Geometry check sheet. Reference: the model listing, model coordinates, mm. A direction names the side the tool comes from. Round coordinates to 2 decimals unless told otherwise and drop trailing zeros. Order: outer loops, then holes, each group sorted by start corner. A loop starts at its lowest first (then second) coordinate and runs counter-clockwise, first axis right, second up.
(1) Thickness scan on L1, parallel to Z at x = 1.25, y = 29; L2, parallel to X at y = 22, z = 0; L3, parallel to Y at x = -1.5, z = -1.5. Record the ranges inside material, lowest first.
(2) Draft check along X on faces 1 (the face through (-0.7, 43, 2.3)), 2 (the face through (-2.44, 19.72, -0.54)), 3 (the face through (-1.07, 42.01, -1.88)). Enter one of: pulls with the +X half, pulls with the -X half, needs draft (parallel to the pull), parting line crosses it, or undercut.
(3) Cross-section at B-B on y = 23. Enter the section's corners in (x, z).
(4) Gauge pin test, flat ends, axial feed: P1, Ø3.5, axis at x = 0, z = 0, coming from the +Y side; P2, Ø3, axis at x = -2, z = 1, coming from the +Y side; P3, Ø4, axis at x = 2.5, y = 25.5, coming from the -Z side. Record the tip position at first contact, or that the pin passes through.
(5) Set-up check for faces 4 (the face through (-3.417, 41.986, -0.759)), 5 (the face through (1.098, 42.014, -1.866)): record each of +Z, -Z, +X, -X, +Y, -Y from which the full face is reachable in a straight line by a thin tool's end or side.
from build123d import *

# Parameters (mm, degrees)
SKETCH1_R          = 2.5
SCREW_LENGTH_DEPTH = 40
SKETCH2_R          = 3.5
SCREW_CAP_DEPTH    = 3
SCREW_HOLE_DEPTH   = 2
CHAMFER1_SIZE      = 1


with BuildPart() as part:
    # Sketch1 → Screw Length (new body)
    with BuildSketch(Plane(origin=(0, 0, 0), x_dir=(1, 0, 0), z_dir=(0, 1, 0))):
        with Locations(Location((0, 0, 0), (0, 0, 270))):
            Circle(SKETCH1_R)
    extrude(amount=SCREW_LENGTH_DEPTH)

    # Sketch2 → Screw Cap (add)
    with BuildSketch(Plane(origin=(0, 40, 0), x_dir=(1, 0, 0), z_dir=(0, 1, 0))):
        with Locations(Location((0, 0, 0), (0, 0, 270))):
            Circle(SKETCH2_R)
    extrude(amount=SCREW_CAP_DEPTH)

    # Sketch3 → Screw Hole (cut)
    with BuildSketch(Plane(origin=(0, 43, 0), x_dir=(1, 0, 0), z_dir=(0, 1, 0))):
        Polygon((0, 2.5), (-2.165063509, 1.25), (-2.165063509, -1.25), (0, -2.5), (2.165063509, -1.25), (2.165063509, 1.25), align=None)
    extrude(amount=-SCREW_HOLE_DEPTH, mode=Mode.SUBTRACT)

    # Chamfer1
    chamfer1_edges = [part.edges().sort_by_distance(p)[0] for p in [
        (0, 40, -3.5),
    ]]
    chamfer(chamfer1_edges, length=CHAMFER1_SIZE - 0.0001)  # a hair under: the kernel refuses the full size


solid = part.part
Found:
1. L1: z = -2.17 to 2.17
1. L2: x = -2.5 to 2.5
1. L3: y = 0 to 41
2. face 1: needs draft
2. face 2: parting line crosses it
2. face 3: undercut
3. outline: circle Ø5 at (0, 0)
4. P1: stops at y = 41
4. P2: stops at y = 43
4. P3: stops at z = -2.45
5. face 4: +Y, -Y
5. face 5: +Y
